Verification items for this drawing (mm, ordinates from the low corner). Coordinates: 2 decimals unless noted, no trailing zeros. Write each loop counter-clockwise with the first axis right and the second up, starting at its lowest first coordinate (ties: lowest second). Pieces come first, ordered by that corner, then holes. Notation, with made-up numbers: (21, 27) -> (62, 27) arc R24 ccw to (62, 56) -> close; hole circle Ø10 at (50.25, 20.25). An arc over 180 degrees is marked (long way). Put each result on its own line as item: value. Start each with the question number.
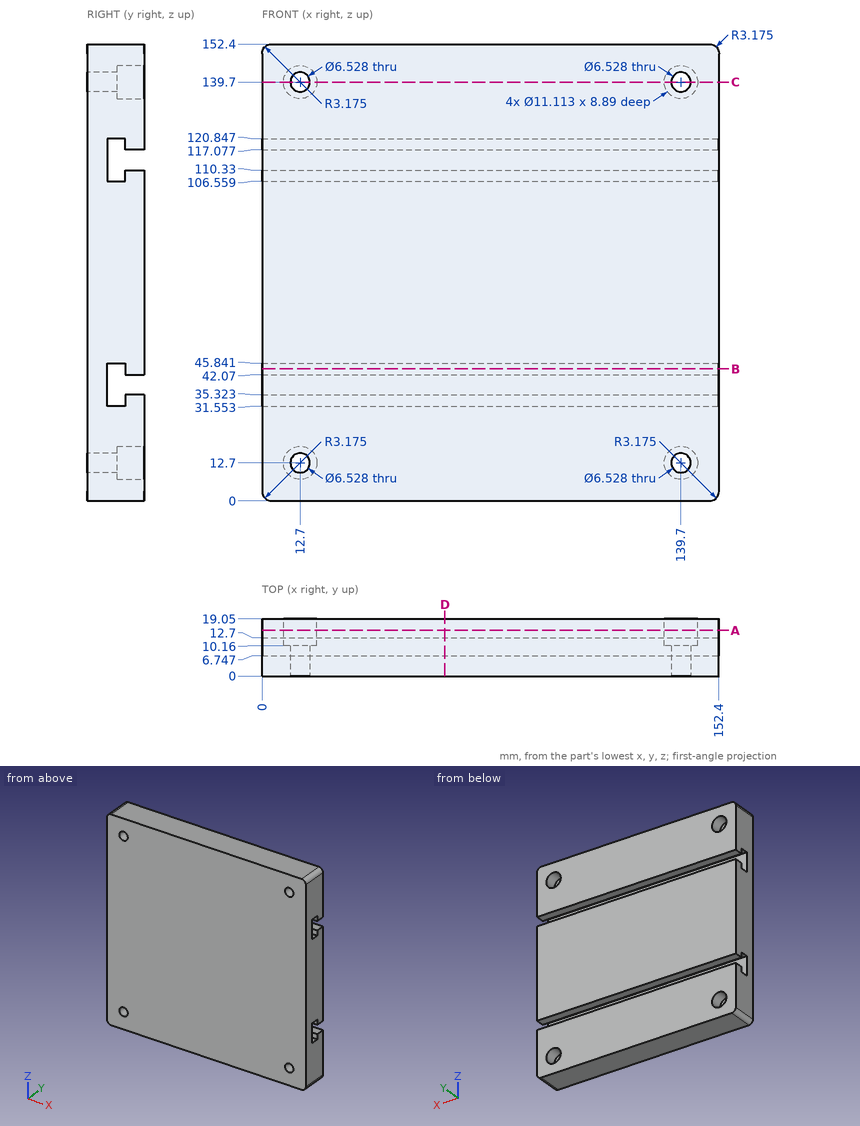
Item 1: Section check D-D, the plane x = 61. Enter the section's corners in (y, z), and give its area (3 significant figures).
Item 2: Section check C-C, the plane z = 139.7. Enter the section's corners in (x, y).
Item 3: Scan lines: line 1 along Z through (x, y) = (12.7, 8); line 2 along X through (y, z) = (16.5, 139.7); line 3 along Z through (x, y) = (139.7, 13.5). Record each from-to range of solid material in increasing order. Write a range as [from, to].
Item 4: Section check A-A, the plane y = 15.25. Give the number of separate pieces and of enclosed holes in the cut face, and give its area (3 significant figures).
Item 5: Section check B-B, the plane z = 44. Enter the section's corners in (x, y), and give its area (3 significant figures).
Item 6: Go/stop test with flat-tipped pins: P1, Ø1.1, axis at x = 39, z = 34, coming from the -Y side; P2, Ø5.5, axis at x = 11, z = 11.5, coming from the +Y side. Record where each tip stops, or that it passes through.
From the geometry:
1. outline: (0, 0) -> (19.05, 0) -> (19.05, 35.32) -> (12.7, 35.32) -> (12.7, 31.55) -> (6.75, 31.55) -> (6.75, 45.84) -> (12.7, 45.84) -> (12.7, 42.07) -> (19.05, 42.07) -> (19.05, 110.33) -> (12.7, 110.33) -> (12.7, 106.56) -> (6.75, 106.56) -> (6.75, 120.85) -> (12.7, 120.85) -> (12.7, 117.08) -> (19.05, 117.08) -> (19.05, 152.4) -> (0, 152.4) -> close
1. area: 2,650 mm²
2. outline: (0, 0) -> (9.44, 0) -> (9.44, 10.16) -> (7.14, 10.16) -> (7.14, 19.05) -> (0, 19.05) -> close; (15.96, 0) -> (136.44, 0) -> (136.44, 10.16) -> (134.14, 10.16) -> (134.14, 19.05) -> (18.26, 19.05) -> (18.26, 10.16) -> (15.96, 10.16) -> close; (142.96, 0) -> (152.4, 0) -> (152.4, 19.05) -> (145.26, 19.05) -> (145.26, 10.16) -> (142.96, 10.16) -> close
3. line 1: [0, 9.44], [15.96, 31.55], [45.84, 106.56], [120.85, 136.44], [142.96, 152.4]
3. line 2: [0, 7.14], [18.26, 134.14], [145.26, 152.4]
3. line 3: [0, 7.14], [18.26, 35.32], [42.07, 110.33], [117.08, 134.14], [145.26, 152.4]
4. separate pieces: 3
4. enclosed holes: 4
4. area: 20,800 mm²
5. outline: (0, 0) -> (152.4, 0) -> (152.4, 6.75) -> (0, 6.75) -> close; (0, 12.7) -> (152.4, 12.7) -> (152.4, 19.05) -> (0, 19.05) -> close
5. area: 2,000 mm²
6. P1: y = 0
6. P2: y = 10.16
